from build123d import *

# Parameters (mm, degrees)
ESQUISSE3_R             = 25
BOSS_EXTRU_2_DEPTH      = 2
ESQUISSE5_R             = 9.75
ESQUISSE5_W             = 3
ESQUISSE5_H             = 4
BOSS_EXTRU_3_DEPTH      = 20
ENL_V_MAT_EXTRU_1_DEPTH = 22
ESQUISSE7_R             = 9.75
BOSS_EXTRU_4_DEPTH      = 3.5
ESQUISSE8_R             = 1.25
ENL_V_MAT_EXTRU_2_DEPTH = 44.591857038
CHANFREIN3_SIZE         = 1
CHANFREIN4_SIZE         = 1
CHANFREIN5_SIZE         = 0.5


with BuildPart() as part:
    # Esquisse3 → Boss.-Extru.2 (new body)
    with BuildSketch(Plane.XY):
        Circle(ESQUISSE3_R)
    extrude(amount=BOSS_EXTRU_2_DEPTH)

    # Esquisse5 → Boss.-Extru.3 (add)
    with BuildSketch(Plane(origin=(0, 0, 0), x_dir=(-1, 0, 0), z_dir=(0, 0, -1))):
        with Locations(Location((0, 0, 0), (0, 0, 180))):
            Circle(ESQUISSE5_R)
        Polygon((-15.216843748, 6.562492138), (-11.412617683, 5.326424161), (-12.339668666, 2.473254612), (-16.143894731, 3.709322589), align=None)
        with Locations((0.039037592, 14.5)):
            Rectangle(ESQUISSE5_W, ESQUISSE5_H)
        Polygon((15.240970307, 6.488238225), (16.16802129, 3.635068676), (12.363795225, 2.399000699), (11.436744242, 5.252170247), align=None)
        Polygon((10.880400079, -12.49004825), (8.453349096, -14.253404007), (6.102208086, -11.017336029), (8.52925907, -9.253980272), align=None)
        Polygon((-8.516513247, -14.207512565), (-10.94356423, -12.444156808), (-8.592423221, -9.20808883), (-6.165372238, -10.971444587), align=None)
    extrude(amount=BOSS_EXTRU_3_DEPTH)

    # Esquisse6 → Enlèv. mat.-Extru.1 (cut)
    with BuildSketch(Plane.XY.offset(2)):
        with BuildLine():
            Line((-2.738612788, 3.25), (2.738612788, 3.25))
            ThreePointArc((2.738612788, 3.25), (0, -4.25), (-2.738612788, 3.25))
        make_face()
    extrude(amount=-ENL_V_MAT_EXTRU_1_DEPTH, mode=Mode.SUBTRACT)

    # Esquisse7 → Boss.-Extru.4 (add)
    with BuildSketch(Plane(origin=(0, 0, -20), x_dir=(-1, 0, 0), z_dir=(0, 0, -1))):
        with Locations(Location((0, 0, 0), (0, 0, 180))):
            Circle(ESQUISSE7_R)
    extrude(amount=BOSS_EXTRU_4_DEPTH)

    # Esquisse8 → Enlèv. mat.-Extru.2 (cut, through all)
    with BuildSketch(Plane(origin=(0, 0, -23.5), x_dir=(-1, 0, 0), z_dir=(0, 0, -1))):
        Circle(ESQUISSE8_R)
    extrude(amount=-ENL_V_MAT_EXTRU_2_DEPTH, mode=Mode.SUBTRACT)

    # Chanfrein3
    chanfrein3_edges = [part.edges().sort_by_distance(p)[0] for p in [
        (14.241781698, 3.091288601, -20),
        (11.876143174, 3.899839386, -20),
        (13.314730715, 5.94445815, -20),
        (15.680369239, 5.135907364, -20),
    ]]
    chamfer(chanfrein3_edges, length=CHANFREIN3_SIZE)

    # Chanfrein4
    chanfrein4_edges = [part.edges().sort_by_distance(p)[0] for p in [
        (-1.539037592, 14.5, -20),
        (-0.039037592, 16.5, -20),
        (1.460962408, 14.5, -20),
        (-0.039037592, 12.5, -20),
        (-14.265908257, 3.017034687, -20),
        (-15.704495798, 5.061653451, -20),
        (-13.338857274, 5.870204236, -20),
        (-11.900269733, 3.825585473, -20),
        (-7.277778591, -12.635370018, -20),
        (-9.666874587, -13.371726128, -20),
        (-9.704829574, -10.872014261, -20),
        (-7.315733578, -10.135658151, -20),
        (9.767993725, -10.826122819, -20),
        (9.730038739, -13.325834686, -20),
        (7.340942742, -12.589478576, -20),
        (7.378897729, -10.089766709, -20),
        (-9.75, 0, -23.5),
    ]]
    chamfer(chanfrein4_edges, length=CHANFREIN4_SIZE)

    # Chanfrein5
    chanfrein5_edges = [part.edges().sort_by_distance(p)[0] for p in [
        (1.25, 0, -20),
    ]]
    chamfer(chanfrein5_edges, length=CHANFREIN5_SIZE)


solid = part.part
Verification items for the finished model (mm, model axes). A direction names the side the tool comes from. Give positions to 0.01 mm unless a question says otherwise; leave off trailing zeros. Order: outer loops, then holes, each group sorted by start corner. A loop starts at its lowest first (then second) coordinate and runs counter-clockwise, first axis right, second up. Notation, with made-up numbers: M 36.5,54 L 93.5,54 A31 ccw 93.5,88 Z; hole C 51.5,41 d4. An arc over 180 degrees is marked long. Answer as a JSON object with one key per item and string values. Group by question number.
1) Depth check by flat-ended pin: pin 1 Ø4 at (x, y) = (-0.5, 0.5) entering from +Z; pin 2 Ø12 at (x, z) = (-17.5, -3) entering from -Y; pin 3 Ø1.7 at (x, y) = (-14.5, 4.5) entering from -Z. Enter the tip coordinate at first touch or a pass-through.
2) Cross-section at D-D (y = 21). Enter the section's corners in (x, z).
3) Cross-section at C-C (y = -20). Enter the section's corners in (x, z).
4) Access from +Z, -Z, +X, -X, +Y, -Y to the whole of each face (thin tool, end or side, straight path). Record for faces 5 (the face through (13.464, 5.577, -19.396)), 6 (the face through (7.324, -12.567, -9.367)), 7 (the face through (15.687, 5.116, -9.367)).
5) Scan lines: line 1 along Y through (x, z) = (0, -9.5); line 2 along Y through (x, z) = (0, -22.5); line 3 along X through (y, z) = (14.5, -18.75). Record each from-to range of solid material in increasing order. Write a range as [from, to].
6) Cross-section at B-B (y = 0). Enter the section's corners in (x, z).
7) Cross-section at A-A (z = -3.75). Enter the section's corners in (x, y), then the cut area to 3 significant figures.
8) Mould release check, pull along Y, two halves, no side actions. Record for faces 1 (the face through (-7.294, -12.658, -9.367)), 2 (the face through (0, 16.5, -9)), 3 (the face through (7.396, -10.077, -9.367)), 4 (the face through (2, -1, -20)): released by +Y, released by -Y, zero draft, split by the parting line, or undercut.
Result sheet:
{
 "1": {"pin 1": "stops at z = -20", "pin 2": "stops at y = -21.76", "pin 3": "stops at z = -20"},
 "2": {"outline": "M -13.56,0 L 13.56,0 L 13.56,2 L -13.56,2 Z"},
 "3": {"outline": "M -15,0 L 15,0 L 15,2 L -15,2 Z"},
 "4": {"face 5": "-Z, +Y", "face 6": "-Z, -Y", "face 7": "-Z, +X, +Y"},
 "5": {"line 1": "y = [-9.75, -4.25], [3.25, 9.75], [12.5, 16.5]", "line 2": "y = [-9.75, -1.25], [1.25, 9.75]", "line 3": "x = [-1.54, 1.46]"},
 "6": {"outline": "M -25,0 L -9.75,0 L -9.75,-22.5 L -8.75,-23.5 L -1.25,-23.5 L -1.25,-20.5 L -1.75,-20 L -4.25,-20 L -4.25,2 L -25,2 Z; M 1.25,-23.5 L 8.75,-23.5 L 9.75,-22.5 L 9.75,0 L 25,0 L 25,2 L 4.25,2 L 4.25,-20 L 1.75,-20 L 1.25,-20.5 Z"},
 "7": {"outline": "M -16.17,3.64 L -12.36,2.4 L -11.44,5.25 L -15.24,6.49 Z; M -10.88,-12.49 L -8.45,-14.25 L -6.1,-11.02 L -8.53,-9.25 Z; C 0,0 d19.5; M -1.54,12.5 L 1.46,12.5 L 1.46,16.5 L -1.54,16.5 Z; M 6.17,-10.97 L 8.52,-14.21 L 10.94,-12.44 L 8.59,-9.21 Z; M 11.41,5.33 L 12.34,2.47 L 16.14,3.71 L 15.22,6.56 Z; hole M -2.74,3.25 A4.25 ccw long 2.74,3.25 Z", "area": "306 mm2"},
 "8": {"face 1": "released by -Y", "face 2": "released by +Y", "face 3": "undercut", "face 4": "undercut"}
}
